For this review, use the dimensioned drawing (mm, ordinates from the lowest corner) and the shaded views. Coordinates: 2 decimals unless noted, no trailing zeros. Loops run counter-clockwise (first coordinate to the right, second up) from the corner with the lowest first, then second, coordinate; pieces in that order, holes last. Notation, with made-up numbers: (12.25, 63) - (34.25, 63) arc R26 cw to (34.25, 87) - close; hole circle Ø8 at (-30.5, 45.5). An arc over 180 degrees is marked (long way). Use one line per item in the form item = value. Start each with the question number.
(1) Add section A-A (z = 1.55). State the section outline as (x, y) points, plus the area to 3 significant figures.
(2) Clearance check with flat-ended pins moving along their axes: pin 1 Ø1.5 at (x, z) = (3, 0.5) entering from -Y; pin 2 Ø1.5 at (y, z) = (3.5, 3) entering from -X; pin 3 Ø1 at (y, z) = (9, 3) entering from +X. State where each tip first meets the part, or that it passes through.
(3) For L1, parallel to Y at x = 7, z = 2.4; L2, parallel to Y at x = 7.75, z = 2.7; L3, parallel to X at y = 5, z = 2.75, list the stretches that pass through material, from the lowest coordinate up.
(4) The part is to be moulded in two halves that separate along X. For the marked faces 1, 2 and 3, say which applies: pulls with the +X half, pulls with the -X half, needs draft (parallel to the pull), parting line crosses it, or undercut.
(5) Add section B-B (z = 0.7). State the section outline as (x, y) points, plus the area to 3 significant figures.
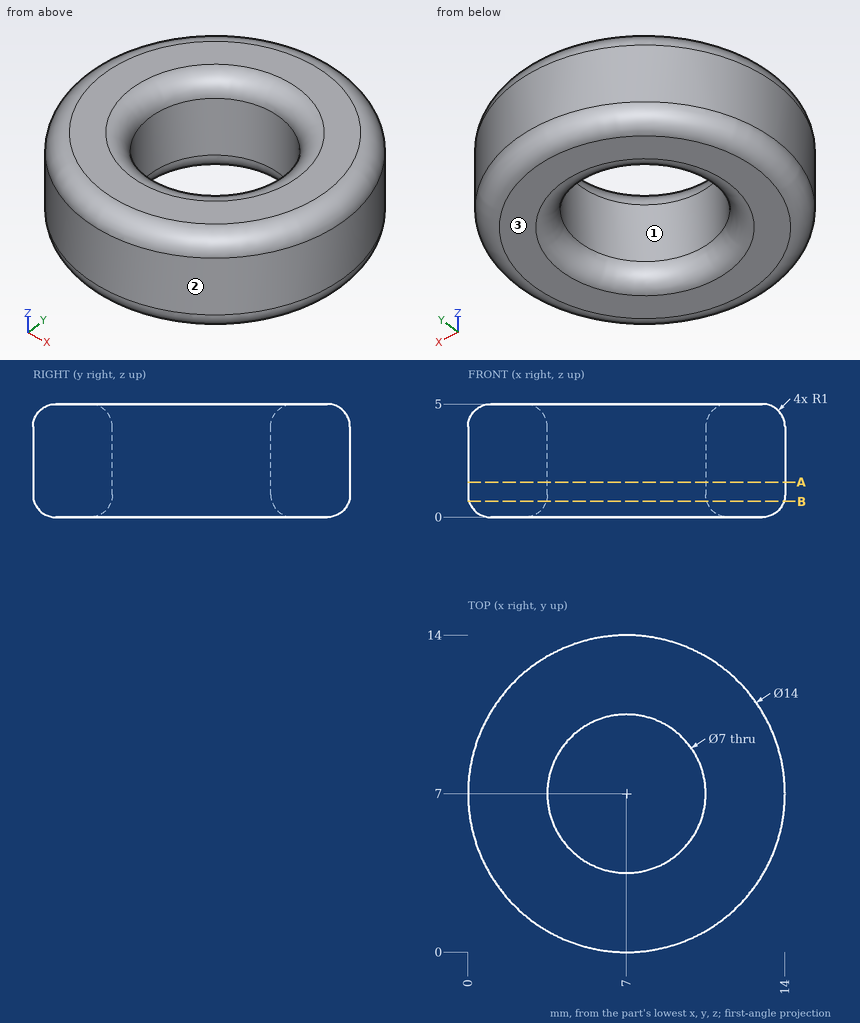
Computed values:
q1.outline = circle Ø14 at (7, 7); hole circle Ø7 at (7, 7)
q1.area = 115 mm^2
q2.pin_1 = 0.86
q2.pin_2 = 0.56
q2.pin_3 = 13.84
q3.L1 = 0 to 3.5, 10.5 to 14
q3.L2 = 0.04 to 3.58, 10.42 to 13.96
q3.L3 = 0.29 to 4.13, 9.87 to 13.71
q4.face_1 = undercut
q4.face_2 = parting line crosses it
q4.face_3 = needs draft
q5.outline = circle Ø13.91 at (7, 7); hole circle Ø7.09 at (7, 7)
q5.area = 112 mm^2
